Read the model definition and answer for the solid it produces. Units are mm, in the model's axes. Face numbers are marked on the shaded views. A direction names the side the tool comes from. Give positions to 0.01 mm unless a question says otherwise; leave off trailing zeros. Loops run counter-clockwise (first coordinate to the right, second up) from the corner with the lowest first, then second, coordinate; pieces in that order, holes last. Notation, with made-up numbers: (-8, -33.75) -> (26, -33.75) arc R28 ccw to (26, -2.75) -> close; hole circle Ø4 at (39, 8.25). An arc over 180 degrees is marked (long way). Write each question's results on one line, items separated by ' | '. Start each with the question number.
Item 1: Which of the six approach directions +Z, -Z, +X, -X, +Y, -Y give full straight-line access (tool end or side, diameter ignored) to the marked faces 1 and 2?
Item 2: Section C-C on x = 8.5 is taken. Write down the section's boundary in (y, z).
Item 3: Each of these flat-tipped pins is pushed along its axis until it touches: P1, Ø2, axis at x = 10, z = 27.5, coming from the +Y side; P2, Ø2.5, axis at y = 7.5, z = 5, coming from the +X side; P3, Ø6, axis at x = 12, z = 22, coming from the -Y side; P4, Ø5, axis at x = 17, y = 9.5, coming from the -Z side. Where does it stop, or does it pass through?
Item 4: Section D-D on y = 15.5 is taken. Write down the section's boundary in (x, z), and give its area (3 significant figures).
Item 5: Section A-A on y = 8.5 is taken. Write down the section's boundary in (x, z).
Item 6: Find the intervals of material crossed by line 1 (X direction, y = 12, z = 5.5); line 2 (X direction, y = 8.75, z = 29); line 3 (Z direction, x = 5.75, y = 11.5), in increasing order.
Item 7: Section B-B on x = 24 is taken. Write down the section's boundary in (y, z).
Autodesk Fusion 360 part; units mm, degrees
sketch "base" plane through (0, 0, 0) normal (0, 0, 1) x (1, 0, 0)
  line L0 (0, 0) -> (18, 0)
  line L1 (18, 0) -> (18, 17)
  line L2 (18, 17) -> (0, 17)
  line L3 (0, 17) -> (0, 0)
  dimension "d1" = 17
  dimension "d2" = 18
extrude "Extrude1" add sketch "base" along normal blind 8
sketch "pins" plane through (18, 0, 0) normal (1, 0, 0) x (0, 1, 0)
  line L0 (0, 0) -> (17, 0)
  line L1 (17, 0) -> (17, 8)
  line L2 (17, 8) -> (0, 8)
  line L3 (0, 8) -> (0, 0)
  circle A0 centre (1.5, 1.5) radius 0.75
  circle A1 centre (8.5, 1.5) radius 0.75
  circle A2 centre (15.5, 1.5) radius 0.75
  dimension "d5" = 1.5
  dimension "d6" = 1.5
  dimension "d7" = 1.5
  dimension "d12" = 14
  dimension "d13" = 0
extrude "Extrude3" add sketch "pins" along normal blind 8 contours A0 | A1 | A2
sketch "base knob" plane through (0, 0, 8) normal (0, 0, 1) x (-1, 0, 0)
  line L0 (0, -17) -> (0, 0)
  line L1 (0, 0) -> (-18, 0)
  line L2 (-18, 0) -> (-18, -17)
  line L3 (-18, -17) -> (0, -17)
  circle A0 centre (-8.5, -8.5) radius 5
  dimension "d16" = 10
  dimension "d17" = 8.5
  dimension "d18" = 8.5
extrude "Extrude4" add sketch "base knob" along normal blind 9 contours A0
sketch "knob" plane through (0, 0, 17) normal (0, 0, 1) x (-1, 0, 0)
  circle A0 centre (-8.5, -8.5) radius 5
  circle A1 centre (-8.5, -8.5) radius 3
  dimension "d21" = 6
extrude "Extrude5" add sketch "knob" along normal blind 35 contours A1
equation "d18 = d17"
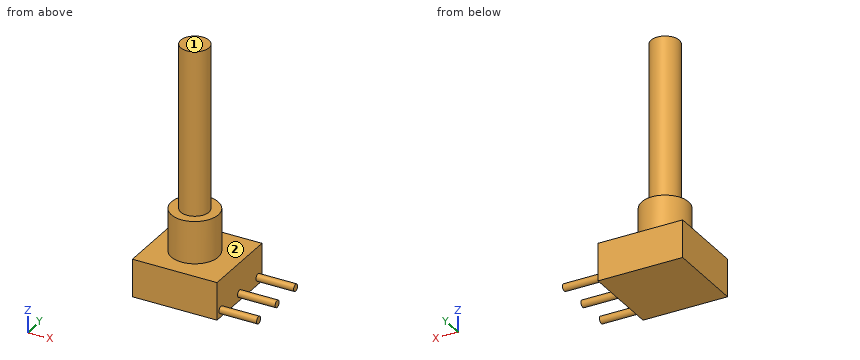
Findings:
1) face 1: +Z, +X, -X, +Y, -Y | face 2: +Z
2) outline: (0, 0) -> (17, 0) -> (17, 8) -> (13.5, 8) -> (13.5, 17) -> (11.5, 17) -> (11.5, 52) -> (5.5, 52) -> (5.5, 17) -> (3.5, 17) -> (3.5, 8) -> (0, 8) -> close
3) P1: y = 11.46 | P2: x = 18 | P3: y = 5.54 | P4: z = 0
4) outline: (0, 0) -> (18, 0) -> (18, 0.75) -> (26, 0.75) -> (26, 2.25) -> (18, 2.25) -> (18, 8) -> (0, 8) -> close | area: 156 mm2
5) outline: (0, 0) -> (18, 0) -> (18, 0.75) -> (26, 0.75) -> (26, 2.25) -> (18, 2.25) -> (18, 8) -> (13.5, 8) -> (13.5, 17) -> (11.5, 17) -> (11.5, 52) -> (5.5, 52) -> (5.5, 17) -> (3.5, 17) -> (3.5, 8) -> (0, 8) -> close
6) line 1: 0 to 18 | line 2: 5.51 to 11.49 | line 3: 0 to 17
7) outline: circle Ø1.5 at (1.5, 1.5); circle Ø1.5 at (8.5, 1.5); circle Ø1.5 at (15.5, 1.5)
